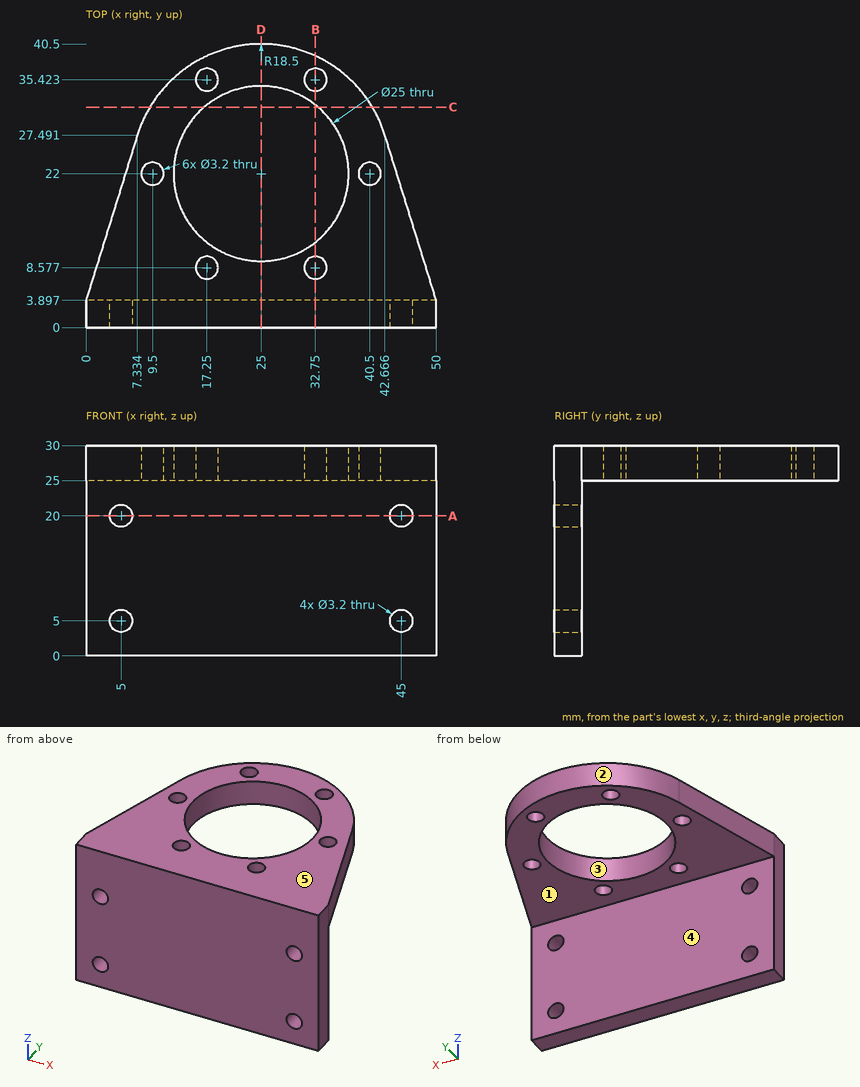
Input: dimensioned drawing with shaded views. Units: mm. Origin: part minimum x, y, z. A direction names the side the tool comes from. Give positions to 0.01 mm unless a question says otherwise; leave off trailing zeros. Order: outer loops, then holes, each group sorted by start corner. A loop starts at its lowest first (then second) coordinate and runs counter-clockwise, first axis right, second up. Notation, with made-up numbers: (-19.75, 57.5) -> (-1.75, 57.5) arc R30 cw to (-1.75, 86.5) -> close; hole circle Ø3 at (48.5, 69). An arc over 180 degrees is marked (long way). Write item = value, one per line.
Item 1: Section query B-B (x = 32.75). Output: boundary loops of the cut face in (y, z).
Check result:
outline = (0, 0) -> (3.9, 0) -> (3.9, 25) -> (6.98, 25) -> (6.98, 30) -> (0, 30) -> close; (10.18, 25) -> (12.19, 25) -> (12.19, 30) -> (10.18, 30) -> close; (31.81, 25) -> (33.82, 25) -> (33.82, 30) -> (31.81, 30) -> close; (37.02, 25) -> (38.8, 25) -> (38.8, 30) -> (37.02, 30) -> close
Item 2: Section query C-C (y = 31.5). Output: boundary loops of the cut face in (x, z) (1 decimal).
Check result:
outline = (9.1, 25) -> (16.9, 25) -> (16.9, 30) -> (9.1, 30) -> close; (33.1, 25) -> (40.9, 25) -> (40.9, 30) -> (33.1, 30) -> close
Item 3: Set-up query: the marked faces 4 and 5. Return all of +Z, -Z, +X, -X, +Y, -Y with unobstructed straight access to the full face (end or side cutting, diameter ignored); none if empty.
Check result:
face_4 = -Z, +X, -X, +Y
face_5 = +Z, +X, -X, +Y, -Y
Item 4: Section query A-A (z = 20). Output: boundary loops of the cut face in (x, y), then the cut area to 3 significant figures.
Check result:
outline = (0, 0) -> (3.4, 0) -> (3.4, 3.9) -> (0, 3.9) -> close; (6.6, 0) -> (43.4, 0) -> (43.4, 3.9) -> (6.6, 3.9) -> close; (46.6, 0) -> (50, 0) -> (50, 3.9) -> (46.6, 3.9) -> close
area = 170 mm²
Item 5: Ray query, probe 1 along Z at (x, y) = (5, 2); probe 2 along Y at (x, z) = (17.25, 28.25) (1 decimal); probe 3 along Y at (x, z) = (3, 3.5). Return the intervals inside material, ascending.
Check result:
probe_1 = 0 to 3.4, 6.6 to 18.4, 21.6 to 30
probe_2 = 0 to 7, 10.2 to 12.2, 31.8 to 33.8, 37 to 38.8
probe_3 = 0 to 3.9
Item 6: Contact query for flat-ended pins moving along their axis: pin 1 (5 mm diameter, centred on x = 23.5, y = 8.5, fed in from -Z); pin 2 (3.5 mm diameter, centred on x = 45, z = 20, fed in from +Y); pin 3 (3 mm diameter, centred on x = 5, z = 5, fed in from -Y) (1 decimal). Output: stop coordinate, or through.
Check result:
pin_1 = 25
pin_2 = 3.9
pin_3 = through
Item 7: Mould query, pull axis X, two halves, no side actions, for the marked faces 1, 2 and 3. Classes: +X half, -X half, draft (parallel to the pull), parting line (faces both ways), or undercut.
Check result:
face_1 = draft
face_2 = parting line
face_3 = undercut
Item 8: Section query D-D (x = 25). Output: boundary loops of the cut face in (y, z).
Check result:
outline = (0, 0) -> (3.9, 0) -> (3.9, 25) -> (9.5, 25) -> (9.5, 30) -> (0, 30) -> close; (34.5, 25) -> (40.5, 25) -> (40.5, 30) -> (34.5, 30) -> close
